Source: three-view drawing plus pictorial views. Frame: mm from the lowest corner of the part. Give positions to 0.01 mm unless a question says otherwise; leave off trailing zeros. Loops run counter-clockwise (first coordinate to the right, second up) from the corner with the lowest first, then second, coordinate; pieces in that order, holes last. Notation, with made-up numbers: (-38.5, -28.5) - (13.5, -28.5) arc R22 cw to (13.5, -12.5) - close; hole circle Ø9 at (47.5, 85). An arc over 180 degrees is marked (long way). Answer as a JSON object with one key per item and string values. Group by question number.
(1) Section query D-D (z = 94.5). Return loops of the section in (x, y).
(2) Section query C-C (x = 30). Return loops of the section in (y, z), plus the area to 3 significant figures.
(3) Section query A-A (y = 7). Count the separate pieces of the cut face and the enclosed holes in it, plus the area to 3 significant figures.
(4) Material intervals for L1, parallel to Z at x = 30, y = 3.25; L2, parallel to X at y = 5.75, z = 94.5; L3, parallel to Z at x = 21, y = 3.25, sorted ascending.
(5) Section query B-B (z = 2.5). Return loops of the section in (x, y).
(6) Pin query (flat end, axial travel): P1, Ø3, axis at x = 30.5, z = 64, coming from the -Y side; P2, Ø12, axis at x = 14, z = 35, coming from the -Y side; P3, Ø1.5, axis at x = 17, y = 3.5, coming from the +Z side. Return the tip coordinate at first contact, or that it passes through.
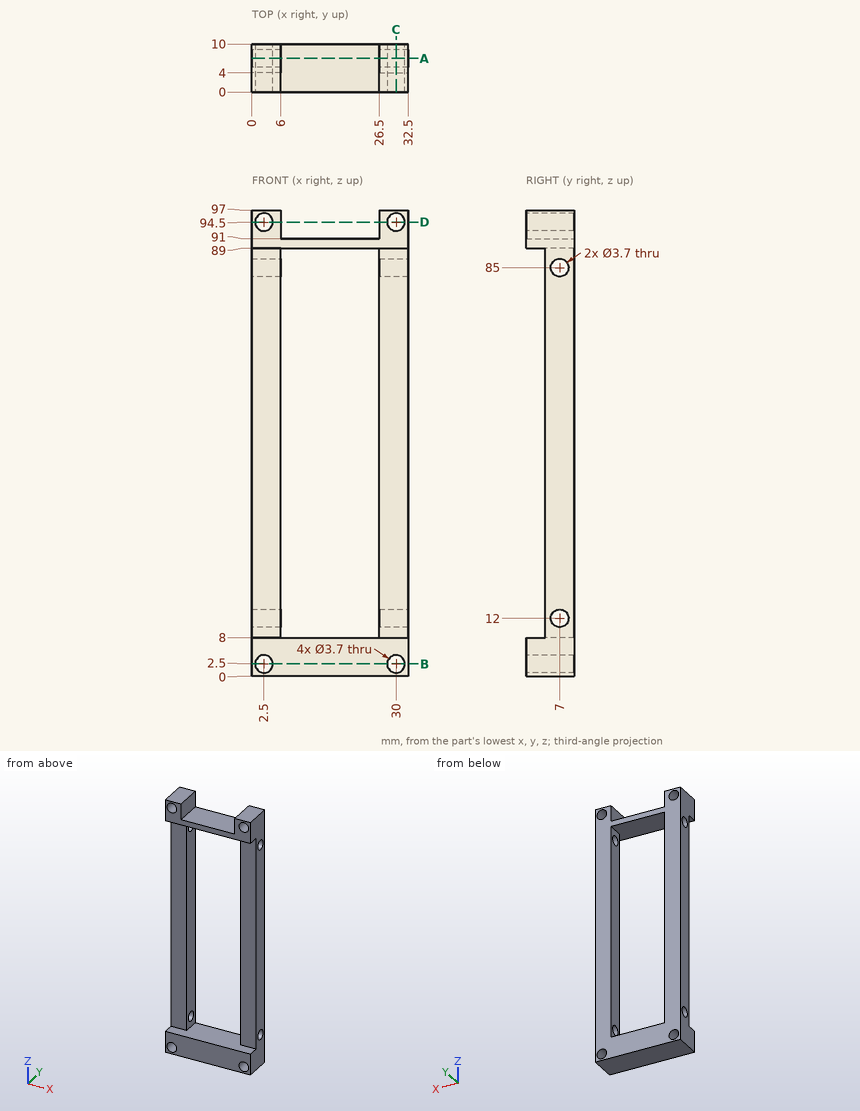
Recorded:
{
 "1": {"outline": "(0, 0) - (0.65, 0) - (0.65, 10) - (0, 10) - close; (4.35, 0) - (6, 0) - (6, 10) - (4.35, 10) - close; (26.5, 0) - (28.15, 0) - (28.15, 10) - (26.5, 10) - close; (31.85, 0) - (32.5, 0) - (32.5, 10) - (31.85, 10) - close"},
 "2": {"outline": "(0, 0) - (10, 0) - (10, 0.65) - (0, 0.65) - close; (0, 4.35) - (10, 4.35) - (10, 92.65) - (0, 92.65) - (0, 89) - (4, 89) - (4, 8) - (0, 8) - close; (0, 96.35) - (10, 96.35) - (10, 97) - (0, 97) - close; hole circle Ø3.7 at (7, 12); hole circle Ø3.7 at (7, 85)", "area": "550 mm^2"},
 "3": {"separate pieces": "4", "enclosed holes": "4", "area": "1,240 mm^2"},
 "4": {"L1": "z = 0 to 0.65, 4.35 to 8, 89 to 92.65, 96.35 to 97", "L2": "x = 0 to 0.65, 4.35 to 6, 26.5 to 28.15, 31.85 to 32.5", "L3": "z = 0 to 8, 89 to 91"},
 "5": {"outline": "(0, 0) - (0.65, 0) - (0.65, 10) - (0, 10) - close; (4.35, 0) - (28.15, 0) - (28.15, 10) - (4.35, 10) - close; (31.85, 0) - (32.5, 0) - (32.5, 10) - (31.85, 10) - close"},
 "6": {"P1": "stops at y = 4", "P2": "passes through", "P3": "stops at z = 91"}
}
